```python
from build123d import *

# Parameters (mm, degrees)
F0_W      = 38.1
F0_H      = 38.1
F1_DEPTH  = 38.1
F6_DEPTH  = 38.1
F8_DEPTH  = 38.1
F9_W      = 25.4
F9_H      = 7.62
F10_DEPTH = 38.1


with BuildPart() as f1:
    # F0 (on Front) → F1 (new body)
    with BuildSketch(Plane.XZ):
        with Locations((19.05, 19.05)):
            Rectangle(F0_W, F0_H)
    extrude(amount=F1_DEPTH)

    # F5 (on offset) → F6 (cut)
    with BuildSketch(Plane.YZ.offset(38.1)):
        Polygon((-11.43, 15.013679), (-6.35, 38.1), (-31.75, 38.1), (-26.67, 17.235135), (-21.59, 28.575), (-16.51, 28.575), align=None)
        Polygon((0, 0), (0, 38.1), (-6.35, 0), align=None)
        Polygon((-25.4, 0), (-12.7, 0), (-19.05, 15.875), align=None)
        Polygon((-31.75, 0), (-38.1, 38.1), (-38.1, 0), align=None)
    extrude(amount=-F6_DEPTH, mode=Mode.SUBTRACT)

    # F7 (on offset) → F8 (cut)
    with BuildSketch(Plane.XZ.offset(38.1)):
        Polygon((0, 38.1), (0, 0), (6.35, 38.1), align=None)
        Polygon((25.4, 38.1), (12.7, 38.1), (19.05, 21.709906), align=None)
        Polygon((31.75, 38.1), (38.1, 0), (38.1, 38.1), align=None)
        Polygon((11.43, 22.225), (6.35, 0), (31.75, 0), (26.67, 22.225), (21.59, 9.009906), (16.51, 9.009906), align=None)
    extrude(amount=-F8_DEPTH, mode=Mode.SUBTRACT)

    # F9 (on offset) → F10 (cut)
    with BuildSketch(Plane.XY.offset(38.1)):
        with Locations((12.7, -26.67)):
            Rectangle(F9_W, F9_H)
        with Locations((25.4, -11.43)):
            Rectangle(F9_W, F9_H)
    extrude(amount=-F10_DEPTH, mode=Mode.SUBTRACT)


solid = f1.part
```
For this review, take the finished solid that the model builds, in its own axes (mm). A direction names the side the tool comes from. Round coordinates to 2 decimals unless told otherwise and drop trailing zeros. Loops run counter-clockwise (first coordinate to the right, second up) from the corner with the lowest first, then second, coordinate; pieces in that order, holes last.
(1) We need section C-C (z = 16.5). State how many separate pieces and enclosed holes the cut face has, plus the area to 3 significant figures.
Returned:
separate pieces: 8
enclosed holes: 0
area: 506 mm2
(2) We need section A-A (z = 7). Give the boundary of the cut face in (x, y).
Returned:
outline: (1.17, -32.92) - (7.95, -32.92) - (7.95, -30.48) - (1.17, -30.48) - close; (1.17, -22.86) - (7.95, -22.86) - (7.95, -22.6) - (1.17, -22.6) - close; (1.17, -15.5) - (7.95, -15.5) - (7.95, -5.18) - (1.17, -5.18) - close; (30.15, -32.92) - (36.93, -32.92) - (36.93, -22.6) - (30.15, -22.6) - close; (30.15, -15.5) - (36.93, -15.5) - (36.93, -15.24) - (30.15, -15.24) - close; (30.15, -7.62) - (36.93, -7.62) - (36.93, -5.18) - (30.15, -5.18) - close
(3) Mouldability with a two-part tool opening along Y and no side actions: class faces 4 (the flat face through (28, -19, 28.575)), 5 (the flat face through (19.12, -20.1, 13.25)), 6 (the flat face through (19, -32, 9.01)) as released by +Y, released by -Y, zero draft, split by the parting line, or undercut.
Returned:
face 4: undercut
face 5: undercut
face 6: zero draft
(4) Wall thickness on line 1 along Y through (x, z) = (15, 25.5); line 2 along X through (y, z) = (-22.5, 11) (3 decimals); line 3 along Y through (x, z) = (31, 25.5): over which ranges is each line inside the solid? List them lowest first.
Returned:
line 1: y = -36 to -30.48, -22.86 to -15.36, -7.62 to -2.1
line 2: x = 1.833 to 8.864, 15.745 to 22.355, 29.236 to 36.267
line 3: y = -36 to -28.68, -22.97 to -15.36, -7.62 to -2.1
(5) Clearance check with flat-ended pins moving along their axes: P1, Ø3, axis at x = 30, y = -21, coming from the -Z side; P2, Ø2.5, axis at x = 28.5, y = -19.5, coming from the +Z side (3 decimals); P3, Ø3.5, axis at y = -29.5, z = 22.5, coming from the -X side. State where each tip first meets the part, or that it passes through.
Returned:
P1: stops at z = 7.26
P2: stops at z = 28.575
P3: stops at x = 3.51
(6) Tool access review of faces 1 (the flat face through (13, -30.48, 20)), 2 (the flat face through (5.06, -15.83, 7.83)), 3 (the flat face through (15.83, -33.5, 30.02)): name each direction out of +Z, -Z, +X, -X, +Y, -Y from which nothing blocks a thin tool from reaching the whole face with its end or side.
Returned:
face 1: +Z, -Z, -X
face 2: -Z, +X, -X
face 3: +Z, +Y, -Y
